from build123d import *

# Parameters (mm, degrees)
F0_R     = 36.5125
F0_R_2   = 7
F2_DEPTH = 2
F3_DEPTH = 37
F0_R_3   = 3.3
F4_DEPTH = 8
F5_DEPTH = 65


with BuildPart() as f2:
    # F0 (on Front) → F2 (new body)
    with BuildSketch(Plane.XZ):
        Circle(F0_R)
        Circle(F0_R_2, mode=Mode.SUBTRACT)
    extrude(amount=F2_DEPTH)

    # F0 (on Front) → F3 (join)
    with BuildSketch(Plane.XZ):
        Circle(F0_R_2)
    extrude(amount=F3_DEPTH)



with BuildPart() as f4:
    # F0 (on Front) → F4 (new body)
    with BuildSketch(Plane.XZ):
        with BuildLine():
            ThreePointArc((42.925, 37.425), (41.314087, 41.314087), (37.425, 42.925))
            Line((37.425, 42.925), (-37.425, 42.925))
            ThreePointArc((-37.425, 42.925), (-41.314087, 41.314087), (-42.925, 37.425))
            Line((-42.925, 37.425), (-42.925, -37.425))
            ThreePointArc((-42.925, -37.425), (-41.314087, -41.314087), (-37.425, -42.925))
            Line((-37.425, -42.925), (37.425, -42.925))
            ThreePointArc((37.425, -42.925), (41.314087, -41.314087), (42.925, -37.425))
            Line((42.925, -37.425), (42.925, 37.425))
        make_face()
        with Locations((-34.75, -34.75)):
            Circle(F0_R_3, mode=Mode.SUBTRACT)
        with Locations((34.75, -34.75)):
            Circle(F0_R_3, mode=Mode.SUBTRACT)
        with Locations((-34.75, 34.75)):
            Circle(F0_R_3, mode=Mode.SUBTRACT)
        Circle(F0_R, mode=Mode.SUBTRACT)
        with Locations((34.75, 34.75)):
            Circle(F0_R_3, mode=Mode.SUBTRACT)
        Circle(F0_R)
        Circle(F0_R_2, mode=Mode.SUBTRACT)
    extrude(amount=-F4_DEPTH)


with BuildPart() as f2_1:
    add(f2.part)

    add(f4.part)  # F5 merges F4
    # F1 (on Front) → F5 (join)
    with BuildSketch(Plane.XZ):
        with BuildLine():
            ThreePointArc((29.05, 38.325), (27.702691, 41.577691), (24.45, 42.925))
            Line((24.45, 42.925), (-24.45, 42.925))
            ThreePointArc((-24.45, 42.925), (-27.702691, 41.577691), (-29.05, 38.325))
            Line((-29.05, 38.325), (-29.05, 34.95))
            ThreePointArc((-29.05, 34.95), (-30.77807, 30.77807), (-34.95, 29.05))
            Line((-34.95, 29.05), (-38.325, 29.05))
            ThreePointArc((-38.325, 29.05), (-41.577691, 27.702691), (-42.925, 24.45))
            Line((-42.925, 24.45), (-42.925, -24.45))
            ThreePointArc((-42.925, -24.45), (-41.577691, -27.702691), (-38.325, -29.05))
            Line((-38.325, -29.05), (-34.95, -29.05))
            ThreePointArc((-34.95, -29.05), (-30.77807, -30.77807), (-29.05, -34.95))
            Line((-29.05, -34.95), (-29.05, -38.325))
            ThreePointArc((-29.05, -38.325), (-27.702691, -41.577691), (-24.45, -42.925))
            Line((-24.45, -42.925), (24.45, -42.925))
            ThreePointArc((24.45, -42.925), (27.702691, -41.577691), (29.05, -38.325))
            Line((29.05, -38.325), (29.05, -34.95))
            ThreePointArc((29.05, -34.95), (30.77807, -30.77807), (34.95, -29.05))
            Line((34.95, -29.05), (38.325, -29.05))
            ThreePointArc((38.325, -29.05), (41.577691, -27.702691), (42.925, -24.45))
            Line((42.925, -24.45), (42.925, 24.45))
            ThreePointArc((42.925, 24.45), (41.577691, 27.702691), (38.325, 29.05))
            Line((38.325, 29.05), (34.95, 29.05))
            ThreePointArc((34.95, 29.05), (30.77807, 30.77807), (29.05, 34.95))
            Line((29.05, 34.95), (29.05, 38.325))
        make_face()
    extrude(amount=-F5_DEPTH)


solid = f2_1.part
Could you check a few things on this model? Use its own coordinates, in mm. A direction names the side the tool comes from. Give positions to 0.01 mm unless a question says otherwise; leave off trailing zeros. Write each loop counter-clockwise with the first axis right and the second up, starting at its lowest first coordinate (ties: lowest second). Pieces come first, ordered by that corner, then holes. Notation, with made-up numbers: (33, 43.5) -> (58, 43.5) arc R6 ccw to (58, 54.5) -> close; hole circle Ø10 at (43.5, 11.25). An arc over 180 degrees is marked (long way). Answer as a JSON object with one key per item and string values.
Q1. Suppose I cut it at B-B on y = 16. Write out the boundary of the cut face in (x, z) (3 decimals), then the cut area to 3 significant figures.
Taken from the geometry:
{"outline": "(-42.925, -24.45) arc R4.6 ccw to (-38.325, -29.05) -> (-34.95, -29.05) arc R5.9 cw to (-29.05, -34.95) -> (-29.05, -38.325) arc R4.6 ccw to (-24.45, -42.925) -> (24.45, -42.925) arc R4.6 ccw to (29.05, -38.325) -> (29.05, -34.95) arc R5.9 cw to (34.95, -29.05) -> (38.325, -29.05) arc R4.6 ccw to (42.925, -24.45) -> (42.925, 24.45) arc R4.6 ccw to (38.325, 29.05) -> (34.95, 29.05) arc R5.9 cw to (29.05, 34.95) -> (29.05, 38.325) arc R4.6 ccw to (24.45, 42.925) -> (-24.45, 42.925) arc R4.6 ccw to (-29.05, 38.325) -> (-29.05, 34.95) arc R5.9 cw to (-34.95, 29.05) -> (-38.325, 29.05) arc R4.6 ccw to (-42.925, 24.45) -> close", "area": "6,590 mm²"}
Q2. Which directions (+Z, -Z, +X, -X, +Y, -Y) give clear straight access to the entire face, cutting with the end or side of a thin tool? Please do faces 1 (the flat face through (-37, 36, -29.05)), 2 (the cylindrical face through (-41.54, 36.1, 27.74)), 3 (the flat face through (29.05, 36, 37)).
Taken from the geometry:
{"face 1": "-Z, -X, +Y", "face 2": "+Z, -X, +Y", "face 3": "+Z, +X, +Y"}
Q3. Please list where these lines run through material, in increasing order: L1, parallel to Z at x = 34.75, y = 2.5 (3 decimals); L2, parallel to Y at x = -8.5, z = 24.5; L3, parallel to Y at x = 34, z = 19.
Taken from the geometry:
{"L1": "z = -42.925 to -38.05, -31.45 to 31.45, 38.05 to 42.925", "L2": "y = -2 to 65", "L3": "y = 0 to 65"}
Q4. Suppose I cut it at D-D on z = 0. Write out the boundary of the cut face in (x, y) (1 decimal), then the cut area to 3 significant figures.
Taken from the geometry:
{"outline": "(-42.9, 0) -> (-36.5, 0) -> (-36.5, -2) -> (-7, -2) -> (-7, -37) -> (7, -37) -> (7, -2) -> (36.5, -2) -> (36.5, 0) -> (42.9, 0) -> (42.9, 65) -> (-42.9, 65) -> close", "area": "6,220 mm²"}
Q5. Will these pins go through, and if not, where does the flat tip stop? pin 1 Ø4 at (y, z) = (51.5, -30.5) entering from -X; pin 2 Ø7.5 at (x, z) = (34.75, -34.75) entering from -Y; pin 3 Ø12 at (x, z) = (-25.5, -23) entering from -Y; pin 4 Ø15 at (x, z) = (-29.5, -36.5) entering from +Y.
Taken from the geometry:
{"pin 1": "stops at x = -40.51", "pin 2": "stops at y = 0", "pin 3": "stops at y = -2", "pin 4": "stops at y = 65"}
Q6. Suppose I cut it at A-A on z = 33. Write out the boundary of the cut face in (x, y) (3 decimals).
Taken from the geometry:
{"outline": "(-42.925, 0) -> (-37.548, 0) -> (-37.548, 8) -> (-42.925, 8) -> close; (-31.952, 0) -> (-15.626, 0) -> (-15.626, -2) -> (15.626, -2) -> (15.626, 0) -> (31.952, 0) -> (31.952, 8) -> (29.382, 8) -> (29.382, 65) -> (-29.382, 65) -> (-29.382, 8) -> (-31.952, 8) -> close; (37.548, 0) -> (42.925, 0) -> (42.925, 8) -> (37.548, 8) -> close"}
Q7. Suppose I cut it at C-C on x = -22. Write out the boundary of the cut face in (y, z) (3 decimals).
Taken from the geometry:
{"outline": "(-2, -29.14) -> (0, -29.14) -> (0, -42.925) -> (65, -42.925) -> (65, 42.925) -> (0, 42.925) -> (0, 29.14) -> (-2, 29.14) -> close"}
Q8. We'd pull the mould along Z, two halves only. Please class faces 4 (the cylindrical face through (36.524, 3.944, 37.533)), 5 (the flat face through (42.925, 32, -1)), 6 (the cylindrical face through (41.36, 3.94, 41.27)), 7 (the cylindrical face through (-41.61, 36.1, -27.67)): released by +Z, released by -Z, zero draft, split by the parting line, or undercut.
Taken from the geometry:
{"face 4": "undercut", "face 5": "zero draft", "face 6": "released by +Z", "face 7": "released by -Z"}
